Input: part model. Units: mm. Frame: model coordinates. A direction names the side the tool comes from. Coordinates: 2 decimals unless noted, no trailing zeros. Order: outer loops, then holes, each group sorted by start corner. A loop starts at its lowest first (then second) coordinate and runs counter-clockwise, first axis right, second up. Notation, with made-up numbers: M 56.5,39.25 L 104.5,39.25 A33 cw 104.5,68.25 Z; hole C 84,-39 d5. An arc over 180 degrees is marked long. One line per item, written item: value.
```python
from build123d import *

# Parameters (mm, degrees)
SKETCH2_W           = 125
SKETCH2_H           = 125
BOSS_EXTRUDE1_DEPTH = 200
SHELL1_T            = -5
SKETCH4_W           = 135
SKETCH4_H           = 135
SKETCH4_W_2         = 125
SKETCH4_H_2         = 125
BOSS_EXTRUDE2_DEPTH = 5
SKETCH3_W           = 135
SKETCH3_H           = 135
SKETCH3_W_2         = 125
SKETCH3_H_2         = 125
BOSS_EXTRUDE4_DEPTH = 5


with BuildPart() as part:
    # Sketch2 → Boss-Extrude1 (new body)
    with BuildSketch(Plane.XY):
        Rectangle(SKETCH2_W, SKETCH2_H)
    extrude(amount=BOSS_EXTRUDE1_DEPTH)

    # Shell1
    shell1_openings = [part.faces().sort_by_distance(p)[0] for p in [
        (0, 0, 200),
        (0, 0, 0),
    ]]
    offset(amount=SHELL1_T, openings=shell1_openings, kind=Kind.INTERSECTION)

    # Sketch4 → Boss-Extrude2 (add)
    with BuildSketch(Plane.XY.offset(200)):
        Rectangle(SKETCH4_W, SKETCH4_H)
        Rectangle(SKETCH4_W_2, SKETCH4_H_2, mode=Mode.SUBTRACT)
    extrude(amount=-BOSS_EXTRUDE2_DEPTH)

    # Sketch3 → Boss-Extrude4 (add)
    with BuildSketch(Plane(origin=(0, 0, 0), x_dir=(-1, 0, 0), z_dir=(0, 0, -1))):
        Rectangle(SKETCH3_W, SKETCH3_H)
        Rectangle(SKETCH3_W_2, SKETCH3_H_2, mode=Mode.SUBTRACT)
    extrude(amount=-BOSS_EXTRUDE4_DEPTH)


solid = part.part
```
(1) Draft query along Z for faces 1 (the flat face through (-1, 62.5, 99)), 2 (the flat face through (67.5, -1, 198)), 3 (the flat face through (59, 1, 200)). Return one class per face: released by +Z, released by -Z, zero draft, split by the parting line, or undercut.
Data:
face 1: undercut
face 2: zero draft
face 3: released by +Z
(2) Ray query, line 1 (X direction, y = 20, z = 182.5). Return the intervals inside material, ascending. Write a range as from..to.
Data:
line 1: x = -62.5..-57.5, 57.5..62.5
(3) Access query for faces 4 (the flat face through (-1, -57.5, 99)), 5 (the flat face through (-62.5, -1, 99)), 6 (the flat face through (5, -65, 5)). Directions: +Z, -Z, +X, -X, +Y, -Y. A direction counts if a zero-diameter tool reaches every point of the face in a straight line with its end or side. Return the directions, or none.
Data:
face 4: +Z, -Z
face 5: -X, +Y, -Y
face 6: none
(4) Cut plane A-A on y = 44. Output: boundary loops of the cut face in (x, z).
Data:
outline: M -67.5,0 L -57.5,0 L -57.5,200 L -67.5,200 L -67.5,195 L -62.5,195 L -62.5,5 L -67.5,5 Z; M 57.5,0 L 67.5,0 L 67.5,5 L 62.5,5 L 62.5,195 L 67.5,195 L 67.5,200 L 57.5,200 Z
(5) First-contact query: pin 1 (3 mm diameter, centred on x = -17.5, z = 163.5, fed in from +Y); pin 2 (2 mm diameter, centred on y = 6, z = 146, fed in from +X); pin 3 (4 mm diameter, centred on y = -45.5, z = 73, fed in from -X). Flat tips, straight axial feed; report the tip coordinate or a pass-through.
Data:
pin 1: stops at y = 62.5
pin 2: stops at x = 62.5
pin 3: stops at x = -62.5
(6) Cut plane C-C on z = 96. Output: boundary loops of the cut face in (x, y).
Data:
outline: M -62.5,-62.5 L 62.5,-62.5 L 62.5,62.5 L -62.5,62.5 Z; hole M -57.5,-57.5 L 57.5,-57.5 L 57.5,57.5 L -57.5,57.5 Z
